Check sheet for the modelled part. Datum: model origin and axes. Units: mm. Face numbers are marked on the shaded views. A direction names the side the tool comes from. Coordinates: 2 decimals unless noted, no trailing zeros. Loops run counter-clockwise (first coordinate to the right, second up) from the corner with the lowest first, then second, coordinate; pieces in that order, holes last.
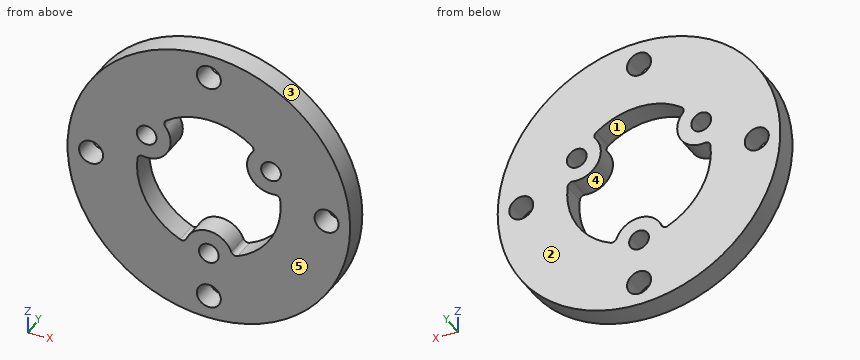
from build123d import *

# Parameters (mm, degrees)
SKETCH1_R           = 30
SKETCH1_R_2         = 10
SKETCH1_R_3         = 2.1
SKETCH1_R_4         = 2.55
BOSS_EXTRUDE1_DEPTH = 5
CUT_EXTRUDE1_DEPTH  = 6
FILLET1_R           = 1


with BuildPart() as part:
    # Sketch1 → Boss-Extrude1 (new body)
    with BuildSketch(Plane(origin=(0, 0, 0), x_dir=(1, 0, 0), z_dir=(0, 1, 0))):
        Circle(SKETCH1_R)
        Circle(SKETCH1_R_2, mode=Mode.SUBTRACT)
        with Locations((0, 15.25)):
            Circle(SKETCH1_R_3, mode=Mode.SUBTRACT)
        with Locations((13.206887408, -7.625)):
            Circle(SKETCH1_R_3, mode=Mode.SUBTRACT)
        with Locations((-13.206887408, -7.625)):
            Circle(SKETCH1_R_3, mode=Mode.SUBTRACT)
        with Locations((0, 25)):
            Circle(SKETCH1_R_4, mode=Mode.SUBTRACT)
        with Locations((25, 0)):
            Circle(SKETCH1_R_4, mode=Mode.SUBTRACT)
        with Locations((0, -25)):
            Circle(SKETCH1_R_4, mode=Mode.SUBTRACT)
        with Locations((-25, 0)):
            Circle(SKETCH1_R_4, mode=Mode.SUBTRACT)
    extrude(amount=BOSS_EXTRUDE1_DEPTH)

    # Sketch2 → Cut-Extrude1 (cut, through all)
    with BuildSketch(Plane(origin=(0, 5, 0), x_dir=(1, 0, 0), z_dir=(0, 1, 0))):
        with BuildLine():
            ThreePointArc((-5.028195952, 14.397213115), (0, 10.15), (5.028195952, 14.397213115))
            ThreePointArc((5.028195952, 14.397213115), (13.206887408, 7.625), (14.982450277, -2.844061128))
            ThreePointArc((14.982450277, -2.844061128), (8.790157848, -5.075), (9.954254325, -11.553151987))
            ThreePointArc((9.954254325, -11.553151987), (0, -15.25), (-9.954254325, -11.553151987))
            ThreePointArc((-9.954254325, -11.553151987), (-8.790157848, -5.075), (-14.982450277, -2.844061128))
            ThreePointArc((-14.982450277, -2.844061128), (-13.206887408, 7.625), (-5.028195952, 14.397213115))
        make_face()
    extrude(amount=-CUT_EXTRUDE1_DEPTH, mode=Mode.SUBTRACT)

    # Fillet1
    fillet1_edges = [part.edges().sort_by_distance(p)[0] for p in [
        (-14.982450277, 2.5, 2.844061128),
        (-5.028195952, 2.5, -14.397213115),
        (5.028195952, 2.5, -14.397213115),
        (14.982450277, 2.5, 2.844061128),
        (9.954254325, 2.5, 11.553151987),
        (-9.954254325, 2.5, 11.553151987),
    ]]
    fillet(fillet1_edges, radius=FILLET1_R)


solid = part.part
(1) Gauge pin test, flat end, axial feed: P1, Ø6.5, axis at x = 0, z = -25, coming from the -Y side. Record the tip position at first contact, or that the pin passes through.
(2) Set-up check for the marked faces 1 and 2: record each of +Z, -Z, +X, -X, +Y, -Y from which the full face is reachable in a straight line by a thin tool's end or side.
(3) Section check A-A, the plane x = 0. Enter the section's corners in (y, z).
(4) Draft check along X on the marked faces 3, 4 and 5. Enter one of: pulls with the +X half, pulls with the -X half, needs draft (parallel to the pull), parting line crosses it, or undercut.
(5) Section check B-B, the plane z = 0. Enter the section's corners in (x, y).
(6) Section check D-D, the plane x = 24. Enter the section's corners in (y, z), plus the area to 3 significant figures.
(7) Scan lines: line 1 along X through (y, z) = (2.65, 0); line 2 along X through (y, z) = (2.65, 2); line 3 along Z through (x, y) = (8.5, 0.6). Record each from-to range of solid material in increasing order.
(8) Section check C-C, the plane z = 25. Enter the section's corners in (x, y), plus the area to 3 significant figures.
Determined:
1. P1: stops at y = 0
2. face 1: +Y, -Y
2. face 2: +Z, -Z, +X, -X, +Y
3. outline: (0, -30) - (5, -30) - (5, -27.55) - (0, -27.55) - close; (0, -22.45) - (5, -22.45) - (5, -17.35) - (0, -17.35) - close; (0, -13.15) - (5, -13.15) - (5, -10.15) - (0, -10.15) - close; (0, 15.25) - (5, 15.25) - (5, 22.45) - (0, 22.45) - close; (0, 27.55) - (5, 27.55) - (5, 30) - (0, 30) - close
4. face 3: parting line crosses it
4. face 4: undercut
4. face 5: needs draft
5. outline: (-30, 0) - (-27.55, 0) - (-27.55, 5) - (-30, 5) - close; (-22.45, 0) - (-15.25, 0) - (-15.25, 5) - (-22.45, 5) - close; (15.25, 0) - (22.45, 0) - (22.45, 5) - (15.25, 5) - close; (27.55, 0) - (30, 0) - (30, 5) - (27.55, 5) - close
6. outline: (0, -18) - (5, -18) - (5, -2.35) - (0, -2.35) - close; (0, 2.35) - (5, 2.35) - (5, 18) - (0, 18) - close
6. area: 157 mm2
7. line 1: x = -30 to -27.55, -22.45 to -15.25, 15.25 to 22.45, 27.55 to 30
7. line 2: x = -29.93 to -26.58, -23.42 to -15.08, 15.08 to 23.42, 26.58 to 29.93
7. line 3: z = -28.77 to -12.66, 5.66 to 9.59, 12.66 to 28.77
8. outline: (-16.58, 0) - (-2.55, 0) - (-2.55, 5) - (-16.58, 5) - close; (2.55, 0) - (16.58, 0) - (16.58, 5) - (2.55, 5) - close
8. area: 140 mm2
